Could you check a few things on this model? Use its own coordinates, in mm. A direction names the side the tool comes from. Give positions to 0.01 mm unless a question says otherwise; leave off trailing zeros. Loops run counter-clockwise (first coordinate to the right, second up) from the corner with the lowest first, then second, coordinate; pieces in that order, holes last. Notation, with made-up numbers: M 22.25,-14.5 L 42.25,-14.5 A19 ccw 42.25,-7.5 Z; hole C 89.5,-36 d3. An arc over 180 degrees is marked long. Use a Markdown table: item, result. Add a question column.
1) Which directions (+Z, -Z, +X, -X, +Y, -Y) give clear straight access to the entire face, cutting with the end or side of a thin tool? Please do faces 1 (the flat face through (15.363, 6.83, 2.465)), 2 (the cylindrical face through (14.492, 3.871, 2.465)), 3 (the cylindrical face through (5.39, 14, 2.46)).
2) Suppose I cut it at A-A on x = -5. List the corners of the cut face in (y, z) for me, and give its area (3 significant figures).
3) Suppose I cut it at B-B on x = 6.5. List the corners of the cut face in (y, z) for me, and give its area (3 significant figures).
4) We'd pull the mould along Y, two halves only. Please class faces 4 (the flat face through (8.41, 14.56, 2.46)), 5 (the flat face through (15.88, 0.56, 2.46)), 6 (the cylindrical face through (-2.026, 2.873, 2.535)): +Y half, -Y half, draft (parallel to the pull), parting line (faces both ways), or undercut.
5) If I drill on line 1 along Y through (x, z) = (0, 2.65); line 2 along Y through (x, z) = (-1, 1.05); line 3 along X through (y, z) = (-1.75, 3.3), over which ranges is the centre line in solid material (lowest first)? Write a range as [from, to].
6) Will these pins go through, and if not, where does the flat tip stop? pin 1 Ø1 at (y, z) = (11, 4.5) entering from -X; pin 2 Ø1.5 at (x, z) = (10.5, 2) entering from -Y; pin 3 Ø3 at (y, z) = (8, 4) entering from -X.
```python
from build123d import *

# Parameters (mm, degrees)
SKETCH1_R           = 2.5
BOSS_EXTRUDE1_DEPTH = 5
FILLET1_R           = 2
FILLET2_R           = 2


with BuildPart() as part:
    # Sketch1 → Boss-Extrude1 (new body)
    with BuildSketch(Plane.XY):
        with BuildLine():
            Line((-7.5, 12.990381057), (-1.5, 2.598076211))
            ThreePointArc((-1.5, 2.598076211), (-1.5, -2.598076211), (3, 0))
            Line((3, 0), (15, 0))
            ThreePointArc((15, 0), (14.999991842, 0.01564381), (14.999967369, 0.031287604))
            Line((14.999967369, 0.031287604), (16.788955727, 1.106220256))
            Line((16.788955727, 1.106220256), (16.652072887, 2.408573483))
            Line((16.652072887, 2.408573483), (14.761035736, 3.059709792))
            Line((14.761035736, 3.059709792), (14.678687152, 3.088064683))
            ThreePointArc((14.678687152, 3.088064683), (14.488887394, 3.882285677), (14.25614831, 4.665001112))
            Line((14.25614831, 4.665001112), (15.625404887, 6.24015062))
            Line((15.625404887, 6.24015062), (15.09277229, 7.43646302))
            Line((15.09277229, 7.43646302), (13.0930769, 7.471367833))
            Line((13.0930769, 7.471367833), (13.0059966, 7.472887825))
            ThreePointArc((13.0059966, 7.472887825), (12.580058519, 8.169585525), (12.116838125, 8.842071808))
            Line((12.116838125, 8.842071808), (12.932330549, 10.763251564))
            Line((12.932330549, 10.763251564), (12.056085985, 11.736419743))
            Line((12.056085985, 11.736419743), (10.143476473, 11.151676334))
            Line((10.143476473, 11.151676334), (10.060188482, 11.12621264))
            ThreePointArc((10.060188482, 11.12621264), (9.439805866, 11.657189422), (8.791447401, 12.153618909))
            Line((8.791447401, 12.153618909), (8.973349591, 14.232770453))
            Line((8.973349591, 14.232770453), (7.839265983, 14.887533929))
            Line((7.839265983, 14.887533929), (6.200961894, 13.740381057))
            Line((6.200961894, 13.740381057), (6.129619023, 13.69042624))
            ThreePointArc((6.129619023, 13.69042624), (5.375519243, 14.003706397), (4.605488553, 14.275485112))
            Line((4.605488553, 14.275485112), (4.135994655, 16.309086604))
            Line((4.135994655, 16.309086604), (2.855084007, 16.581352567))
            Line((2.855084007, 16.581352567), (1.651453961, 14.984081547))
            Line((1.651453961, 14.984081547), (1.599039745, 14.914525534))
            ThreePointArc((1.599039745, 14.914525534), (0.785039344, 14.979443021), (-0.031287604, 14.999967369))
            Line((-0.031287604, 14.999967369), (-1.106220256, 16.788955727))
            Line((-1.106220256, 16.788955727), (-2.408573483, 16.652072887))
            Line((-2.408573483, 16.652072887), (-3.059709792, 14.761035736))
            Line((-3.059709792, 14.761035736), (-3.088064683, 14.678687152))
            ThreePointArc((-3.088064683, 14.678687152), (-3.882285677, 14.488887394), (-4.665001112, 14.25614831))
            Line((-4.665001112, 14.25614831), (-6.24015062, 15.625404887))
            Line((-6.24015062, 15.625404887), (-7.43646302, 15.09277229))
            Line((-7.43646302, 15.09277229), (-7.471367833, 13.0930769))
            Line((-7.471367833, 13.0930769), (-7.472887825, 13.0059966))
            ThreePointArc((-7.472887825, 13.0059966), (-7.486447984, 12.998195897), (-7.5, 12.990381057))
        make_face()
        Circle(SKETCH1_R, mode=Mode.SUBTRACT)
    extrude(amount=BOSS_EXTRUDE1_DEPTH)

    # Fillet1
    fillet1_edges = [part.edges().sort_by_distance(p)[0] for p in [
        (-1.5, 2.598076211, 2.5),
    ]]
    fillet(fillet1_edges, radius=FILLET1_R)

    # Fillet2
    fillet2_edges = [part.edges().sort_by_distance(p)[0] for p in [
        (3, 0, 2.5),
    ]]
    fillet(fillet2_edges, radius=FILLET2_R)


solid = part.part
```
Answer block:
| question | item | result |
|---|---|---|
| 1 | face 1 | +Z, -Z, +X, +Y |
| 1 | face 2 | +Z, -Z, +X |
| 1 | face 3 | +Z, -Z, +Y |
| 2 | outline | M 8.66,0 L 14.55,0 L 14.55,5 L 8.66,5 Z |
| 2 | area | 29.4 mm^2 |
| 3 | outline | M 0,0 L 13.95,0 L 13.95,5 L 0,5 Z |
| 3 | area | 69.7 mm^2 |
| 4 | face 4 | +Y half |
| 4 | face 5 | -Y half |
| 4 | face 6 | undercut |
| 5 | line 1 | y = [-3, -2.5], [2.5, 15] |
| 5 | line 2 | y = [-2.83, -2.29], [2.29, 16.61] |
| 5 | line 3 | x = [-2.44, -1.79], [1.79, 2.44] |
| 6 | pin 1 | stops at x = -6.64 |
| 6 | pin 2 | stops at y = 0 |
| 6 | pin 3 | stops at x = -5.48 |
